```python
from build123d import *

# Parameters (mm, degrees)
SKETCH_W                           = 10
SKETCH_H                           = 168
PAD_DEPTH                          = 5
POCKET_DEPTH                       = 2.15
SKETCH002_R                        = 1.7
HOLE_DEPTH                         = 339.594226
POCKET_LINEARPATTERN_2_DEPTH       = 2.15
SKETCH002_LINEARPATTERN_2_R        = 1.7
HOLE_LINEARPATTERN_2_DEPTH         = 339.594226
LINEARPATTERN001_COUNT             = 4
LINEARPATTERN001_PITCH             = 42
SKETCH003_W                        = 168
SKETCH003_H                        = 5
PAD001_DEPTH                       = 20
POCKET001_DEPTH                    = 2.15
SKETCH005_R                        = 1.7
HOLE001_DEPTH                      = 344.312564
POCKET001_LINEARPATTERN002_2_DEPTH = 2.15
SKETCH005_LINEARPATTERN002_2_R     = 1.7
HOLE001_LINEARPATTERN002_2_DEPTH   = 344.312564
LINEARPATTERN003_COUNT             = 5
LINEARPATTERN003_PITCH             = 33.6
FILLET_R                           = 5


with BuildPart() as part:
    # Sketch → Pad (new body)
    with BuildSketch(Plane.XY):
        with Locations((0, -79)):
            Rectangle(SKETCH_W, SKETCH_H)
    extrude(amount=PAD_DEPTH)

    # Sketch001 (on Face6 of Pad) → Pocket (cut)
    with BuildSketch(Plane.XY.offset(5)):
        Polygon((3.348632, 0), (1.674316, 2.9), (-1.674316, 2.9), (-3.348632, 0), (-1.674316, -2.9), (1.674316, -2.9), align=None)
    pocket = extrude(amount=-POCKET_DEPTH, mode=Mode.SUBTRACT)

    # Sketch002 (on Face13 of Pocket) → Hole (cut, through all)
    with BuildSketch(Plane.XY.offset(2.85)):
        Circle(SKETCH002_R)
    hole = extrude(amount=-HOLE_DEPTH, mode=Mode.SUBTRACT)

    # Sketch001 LinearPattern 2 → Pocket LinearPattern 2 (cut)
    with BuildSketch(Plane(origin=(0, -31, 5), x_dir=(1, 0, 0), z_dir=(0, 0, 1))):
        Polygon((3.348632, 0), (1.674316, 2.9), (-1.674316, 2.9), (-3.348632, 0), (-1.674316, -2.9), (1.674316, -2.9), align=None)
    pocket_linearpattern_2 = extrude(amount=-POCKET_LINEARPATTERN_2_DEPTH, mode=Mode.SUBTRACT)

    # Sketch002 LinearPattern 2 → Hole LinearPattern 2 (cut, through all)
    with BuildSketch(Plane(origin=(0, -31, 2.85), x_dir=(1, 0, 0), z_dir=(0, 0, 1))):
        Circle(SKETCH002_LINEARPATTERN_2_R)
    hole_linearpattern_2 = extrude(amount=-HOLE_LINEARPATTERN_2_DEPTH, mode=Mode.SUBTRACT)

    # LinearPattern001: Pocket, Hole, Pocket LinearPattern 2, Hole LinearPattern 2 ×4
    with Locations(*[(0, -i * LINEARPATTERN001_PITCH, 0) for i in range(1, LINEARPATTERN001_COUNT)]):
        add(pocket, mode=Mode.SUBTRACT)
        add(hole, mode=Mode.SUBTRACT)
        add(pocket_linearpattern_2, mode=Mode.SUBTRACT)
        add(hole_linearpattern_2, mode=Mode.SUBTRACT)

    # Sketch003 (on Face2 of MultiTransform) → Pad001 (join)
    with BuildSketch(Plane(origin=(-5, 0, 0), x_dir=(0, -1, 0), z_dir=(-1, 0, 0))):
        with Locations((79, 2.5)):
            Rectangle(SKETCH003_W, SKETCH003_H)
    extrude(amount=PAD001_DEPTH)

    # Sketch004 (on Face7 of Pad001) → Pocket001 (cut)
    with BuildSketch(Plane(origin=(0, 0, 0), x_dir=(1, 0, 0), z_dir=(0, 0, -1))):
        Polygon((-14.151368, 153.7), (-15.825684, 156.6), (-19.174316, 156.6), (-20.848632, 153.7), (-19.174316, 150.8), (-15.825684, 150.8), align=None)
    pocket001 = extrude(amount=-POCKET001_DEPTH, mode=Mode.SUBTRACT)

    # Sketch005 (on Face81 of Pocket001) → Hole001 (cut, through all)
    with BuildSketch(Plane(origin=(0, 0, 2.15), x_dir=(1, 0, 0), z_dir=(0, 0, -1))):
        with Locations((-17.5, 153.7)):
            Circle(SKETCH005_R)
    hole001 = extrude(amount=-HOLE001_DEPTH, mode=Mode.SUBTRACT)

    # Sketch004 LinearPattern002 2 → Pocket001 LinearPattern002 2 (cut)
    with BuildSketch(Plane(origin=(0, 15, 0), x_dir=(1, 0, 0), z_dir=(0, 0, -1))):
        Polygon((-14.151368, 153.7), (-15.825684, 156.6), (-19.174316, 156.6), (-20.848632, 153.7), (-19.174316, 150.8), (-15.825684, 150.8), align=None)
    pocket001_linearpattern002_2 = extrude(amount=-POCKET001_LINEARPATTERN002_2_DEPTH, mode=Mode.SUBTRACT)

    # Sketch005 LinearPattern002 2 → Hole001 LinearPattern002 2 (cut, through all)
    with BuildSketch(Plane(origin=(0, 15, 2.15), x_dir=(1, 0, 0), z_dir=(0, 0, -1))):
        with Locations((-17.5, 153.7)):
            Circle(SKETCH005_LINEARPATTERN002_2_R)
    hole001_linearpattern002_2 = extrude(amount=-HOLE001_LINEARPATTERN002_2_DEPTH, mode=Mode.SUBTRACT)

    # LinearPattern003: Pocket001, Hole001, Pocket001 LinearPattern002 2, Hole001 LinearPattern002 2 ×5
    with Locations(*[(0, i * LINEARPATTERN003_PITCH, 0) for i in range(1, LINEARPATTERN003_COUNT)]):
        add(pocket001, mode=Mode.SUBTRACT)
        add(hole001, mode=Mode.SUBTRACT)
        add(pocket001_linearpattern002_2, mode=Mode.SUBTRACT)
        add(hole001_linearpattern002_2, mode=Mode.SUBTRACT)

    # Fillet
    fillet_edges = [part.edges().sort_by_distance(p)[0] for p in [
        (5, -163, 2.5),
        (-25, -163, 2.5),
        (5, 5, 2.5),
        (-25, 5, 2.5),
    ]]
    fillet(fillet_edges, radius=FILLET_R)


solid = part.part
```
Could you check a few things on this model? Use its own coordinates, in mm. A direction names the side the tool comes from. Coordinates: 2 decimals unless noted, no trailing zeros. Answer as CSV lines item,"result". Start each with the question number.
1) Please list where these lines run through material, in increasing order: line 1 (X direction, y = -84, z = 1.55); line 2 (X direction, y = -38, z = 3.7); line 3 (X direction, y = -40, z = 1.35). Write a range as from..to.
2) For faces 1 (the flat face through (-16, -73, 2.15)), 2 (the flat face through (1.4, -29.7, 2.85)), 3 (the cylindrical face through (-24, -161, 3)), which set-ups out of +Z, -Z, +X, -X, +Y, -Y let a thin tool reach every point of the face, with its end or its side?
3) For P1, Ø4.5, axis at x = -17.5, y = -86.5, coming from the -Z side; P2, Ø2, axis at x = -17.5, y = -105.1, coming from the -Z side; P3, Ø4, axis at x = -0.5, y = -31.5, coming from the +Z side, each with a flat end and sliding along its axis, tell me the tip position at first contact or that it passes through.
4) We'd pull the mould along Y, two halves only. Please class faces 4 (the flat face through (-16, -54, 2.15)), 5 (the cylindrical face through (-23, 4, 3)), 6 (the flat face through (-10, -163, 2)): +Y half, -Y half, draft (parallel to the pull), parting line (faces both ways), or undercut.
5) I want a section at A-A, the plane z = 3.6. Give the number of separate pieces and of enclosed holes in the cut face, and give its area (3 significant figures).
Data:
1,line 1,"x = -25..-19.41, -15.59..-1.7, 1.7..5"
1,line 2,"x = -25..-19.2, -15.8..5"
1,line 3,"x = -25..-19.64, -15.36..5"
2,face 1,"-Z"
2,face 2,"+Z"
2,face 3,"+Z, -Z, -X, -Y"
3,P1,"stops at z = 2.15"
3,P2,"passes through"
3,P3,"stops at z = 2.85"
4,face 4,"undercut"
4,face 5,"+Y half"
4,face 6,"-Y half"
5,separate pieces,"1"
5,enclosed holes,"18"
5,area,"4,690 mm^2"
